Input: part model. Units: mm. Frame: model coordinates. Coordinates: 2 decimals unless noted, no trailing zeros. Write each loop counter-clockwise with the first axis right and the second up, starting at its lowest first coordinate (ties: lowest second). Pieces come first, ordered by that corner, then holes. Notation, with made-up numbers: (18, 33.25) - (40, 33.25) arc R13 cw to (40, 39.25) - close; hole circle Ø6 at (14, -17.5). An arc over 180 degrees is marked (long way). One line per question, with ' | ' between items. Start each with the question number.
1) Line query: line 1 (Y direction, x = 71, z = -1.5); line 2 (Y direction, x = 75.5, z = -0.25); line 3 (X direction, y = 246, z = -0.5). Output: solid intervals per line, ascending.
2) Section query A-A on z = 0.5. Return loops of the section in (x, y) (1 decimal).
3) First-contact query: P1, Ø20.5, axis at x = 65.55, y = 240.07, coming from the -Z side (3 decimals); P2, Ø21, axis at x = 65.55, y = 240.07, coming from the +Z side. Flat tips, straight axial feed; report the tip coordinate or a pass-through.
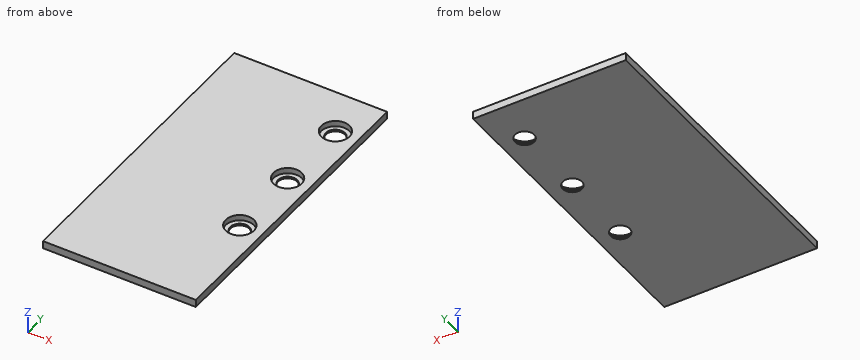
```python
from build123d import *

# Parameters (mm, degrees)
BOSS_EXTRUDE1_DEPTH = 3.175
SKETCH4_R           = 11.7475
CUT_EXTRUDE1_DEPTH  = 4.7625
SKETCH5_R           = 7.9375
CUT_EXTRUDE2_DEPTH  = 2.5875
LPATTERN1_COUNT     = 3
LPATTERN1_PITCH     = 63.5


with BuildPart() as part:
    # Sketch3 → Boss-Extrude1 (new body, symmetric)
    with BuildSketch(Plane(origin=(65.549733265, 163.86644962, 0), x_dir=(1, 0, 0), z_dir=(0, 0, 1))):
        Polygon((19.05, -76.2), (0, -76.2), (-107.95, -76.2), (-107.95, 177.8), (19.05, 177.8), align=None)
    extrude(amount=BOSS_EXTRUDE1_DEPTH, both=True)

    # Sketch4 → Cut-Extrude1 (cut)
    with BuildSketch(Plane.XY.offset(3.175)):
        with Locations((65.549733265, 176.56644962)):
            Circle(SKETCH4_R)
    cut_extrude1 = extrude(amount=-CUT_EXTRUDE1_DEPTH, mode=Mode.SUBTRACT)

    # Sketch5 → Cut-Extrude2 (cut, through all)
    with BuildSketch(Plane.XY.offset(-1.5875)):
        with Locations((65.549733265, 176.56644962)):
            Circle(SKETCH5_R)
    cut_extrude2 = extrude(amount=-CUT_EXTRUDE2_DEPTH, mode=Mode.SUBTRACT)

    # LPattern1: Cut-Extrude1, Cut-Extrude2 ×3
    with Locations(*[(0, i * LPATTERN1_PITCH, 0) for i in range(1, LPATTERN1_COUNT)]):
        add(cut_extrude1, mode=Mode.SUBTRACT)
        add(cut_extrude2, mode=Mode.SUBTRACT)


solid = part.part
```
Answer key:
1) line 1: 87.67 to 166.16, 186.97 to 229.66, 250.47 to 293.16, 313.97 to 341.67 | line 2: 87.67 to 170.32, 182.81 to 233.82, 246.31 to 297.32, 309.81 to 341.67 | line 3: -42.4 to 55.41, 75.69 to 84.6
2) outline: (-42.4, 87.7) - (84.6, 87.7) - (84.6, 341.7) - (-42.4, 341.7) - close; hole circle Ø23.5 at (65.5, 176.6); hole circle Ø23.5 at (65.5, 240.1); hole circle Ø23.5 at (65.5, 303.6)
3) P1: z = -3.175 | P2: z = -1.59
